```python
from build123d import *

# Parameters (mm, degrees)
SKETCH_1_R          = 2
SKETCH_1_R_2        = 4.5
EXTRUDE_1_DEPTH     = 4
SKETCH_4_W          = 70
SKETCH_4_H          = 12
CUT_EXTRUDE_1_DEPTH = 4


with BuildPart() as part:
    # 草图1 → 凸台-拉伸1 (new body)
    with BuildSketch(Plane.XY):
        Polygon((35, 50), (-35, 50), (-35, 41.99755337), (-31, 41.99755337), (-31, 43.29755337), (-28.5, 43.29755337), (-28.5, 41.99755337), (-27, 41.99755337), (-27, 38.99755337), (-28.5, 38.99755337), (-28.5, 37.69755337), (-31, 37.69755337), (-31, 38.99755337), (-35, 38.99755337), (-35, 24.49755337), (-39, 24.49755337), (-39, 16.49755337), (-35, 16.49755337), (-35, 1.99755337), (-31, 1.99755337), (-31, 3.29755337), (-28.5, 3.29755337), (-28.5, 1.99755337), (-27, 1.99755337), (-27, -1.00244663), (-28.5, -1.00244663), (-28.5, -2.30244663), (-31, -2.30244663), (-31, -1.00244663), (-35, -1.00244663), (-35, -15.50244663), (-39, -15.50244663), (-39, -23.50244663), (-35, -23.50244663), (-35, -38.00244663), (-31, -38.00244663), (-31, -36.70244663), (-28.5, -36.70244663), (-28.5, -38.00244663), (-27, -38.00244663), (-27, -41.00244663), (-28.5, -41.00244663), (-28.5, -42.30244663), (-31, -42.30244663), (-31, -41.00244663), (-35, -41.00244663), (-35, -55.50244663), (-39, -55.50244663), (-39, -63.50244663), (-35, -63.50244663), (-35, -87), (35, -87), (35, -63.50244663), (39, -63.50244663), (39, -55.50244663), (35, -55.50244663), (35, -41.00244663), (31, -41.00244663), (31, -42.30244663), (28.5, -42.30244663), (28.5, -41.00244663), (27, -41.00244663), (27, -38.00244663), (28.5, -38.00244663), (28.5, -36.70244663), (31, -36.70244663), (31, -38.00244663), (35, -38.00244663), (35, -23.50244663), (39, -23.50244663), (39, -15.50244663), (35, -15.50244663), (35, -1.00244663), (31, -1.00244663), (31, -2.30244663), (28.5, -2.30244663), (28.5, -1.00244663), (27, -1.00244663), (27, 1.99755337), (28.5, 1.99755337), (28.5, 3.29755337), (31, 3.29755337), (31, 1.99755337), (35, 1.99755337), (35, 16.49755337), (39, 16.49755337), (39, 24.49755337), (35, 24.49755337), (35, 38.99755337), (31, 38.99755337), (31, 37.69755337), (28.5, 37.69755337), (28.5, 38.99755337), (27, 38.99755337), (27, 41.99755337), (28.5, 41.99755337), (28.5, 43.29755337), (31, 43.29755337), (31, 41.99755337), (35, 41.99755337), align=None)
        with Locations((-20, -57)):
            Circle(SKETCH_1_R, mode=Mode.SUBTRACT)
        with Locations((20, -57)):
            Circle(SKETCH_1_R, mode=Mode.SUBTRACT)
        with Locations((-20, -17)):
            Circle(SKETCH_1_R, mode=Mode.SUBTRACT)
        with Locations((0, 3)):
            Circle(SKETCH_1_R, mode=Mode.SUBTRACT)
        with Locations((-20, 23)):
            Circle(SKETCH_1_R, mode=Mode.SUBTRACT)
        with Locations((0, -17)):
            Circle(SKETCH_1_R_2, mode=Mode.SUBTRACT)
        with Locations((20, -17)):
            Circle(SKETCH_1_R, mode=Mode.SUBTRACT)
        with Locations((20, 23)):
            Circle(SKETCH_1_R, mode=Mode.SUBTRACT)
    extrude(amount=EXTRUDE_1_DEPTH)

    # 草图4 → 切除-拉伸1 (cut)
    with BuildSketch(Plane.XY.offset(4)):
        with Locations((0, -81)):
            Rectangle(SKETCH_4_W, SKETCH_4_H)
    extrude(amount=-CUT_EXTRUDE_1_DEPTH, mode=Mode.SUBTRACT)


solid = part.part
```
The model under review builds one solid part; all positions refer to its coordinate system, in mm. A direction names the side the tool comes from. Round coordinates to 2 decimals unless told otherwise and drop trailing zeros. Loops run counter-clockwise (first coordinate to the right, second up) from the corner with the lowest first, then second, coordinate; pieces in that order, holes last. Notation, with made-up numbers: M 54,67 L 90,67 A18 cw 90,102 Z; hole C 12,60.5 d4. An arc over 180 degrees is marked long. Write item = value, one per line.
Item 1: Take a section at C-C on y = -17. Write out the cut boundary in (x, z).
Return value:
outline = M -39,0 L -22,0 L -22,4 L -39,4 Z; M -18,0 L -4.5,0 L -4.5,4 L -18,4 Z; M 4.5,0 L 18,0 L 18,4 L 4.5,4 Z; M 22,0 L 39,0 L 39,4 L 22,4 Z
Item 2: Machinability: for faces 4 (the flat face through (39, 20, 2)), 5 (the flat face through (-39, 21, 2)), 6 (the flat face through (-30, 43.298, 2)), 7 (the flat face through (27, -40, 2)), 8 (the flat face through (-35, -31, 2)), which of the approach directions +Z, -Z, +X, -X, +Y, -Y give a long, thin tool a straight path to every point of the face, cutting with its end or side? Answer none if there is none.
Return value:
face_4 = +Z, -Z, +X, +Y, -Y
face_5 = +Z, -Z, -X, +Y, -Y
face_6 = +Z, -Z
face_7 = +Z, -Z, +X
face_8 = +Z, -Z, -X
Item 3: The part is to be moulded in two halves that separate along Y. For faces 1 (the flat face through (35, 32, 2)), 2 (the flat face through (33, -1.002, 2)), 3 (the flat face through (0, -75, 2)), say which applies: released by +Y, released by -Y, zero draft, split by the parting line, or undercut.
Return value:
face_1 = zero draft
face_2 = undercut
face_3 = released by -Y
Item 4: Take a section at B-B on x = 0. Write out the cut boundary in (y, z), then the cut area to 3 significant figures.
Return value:
outline = M -75,0 L -21.5,0 L -21.5,4 L -75,4 Z; M -12.5,0 L 1,0 L 1,4 L -12.5,4 Z; M 5,0 L 50,0 L 50,4 L 5,4 Z
area = 448 mm2
Item 5: Take a section at D-D on x = 20. Write out the cut boundary in (y, z), then the cut area to 3 significant figures.
Return value:
outline = M -75,0 L -59,0 L -59,4 L -75,4 Z; M -55,0 L -19,0 L -19,4 L -55,4 Z; M -15,0 L 21,0 L 21,4 L -15,4 Z; M 25,0 L 50,0 L 50,4 L 25,4 Z
area = 452 mm2
Item 6: For line 1 (Y direction, x = -20, z = 1.45); line 2 (Y direction, x = 0, z = 2.95); line 3 (X direction, y = -11.5, z = 1), list the stretches that pass through material, from the lowest coordinate up. Write a range as [from, to].
Return value:
line_1 = [-75, -59], [-55, -19], [-15, 21], [25, 50]
line_2 = [-75, -21.5], [-12.5, 1], [5, 50]
line_3 = [-35, 35]
Item 7: Insertion check: P1, Ø0.6, axis at y = -42, z = 1.5, coming from the -X side; P2, Ø2.5, axis at x = -20, y = -17, coming from the +Z side (1 decimal); P3, Ø1.4, axis at y = -1.5, z = 2, coming from the +X side. Each pin has a flat end and moves straight along its axis. Give the tip position at first contact, or say it passes through.
Return value:
P1 = -35
P2 = through
P3 = 35
Item 8: Take a section at A-A on y = 23. Write out the cut boundary in (x, z), then the cut area to 3 significant figures.
Return value:
outline = M -39,0 L -22,0 L -22,4 L -39,4 Z; M -18,0 L 18,0 L 18,4 L -18,4 Z; M 22,0 L 39,0 L 39,4 L 22,4 Z
area = 280 mm2
